Geometry check sheet. Reference: the model listing, model coordinates, mm. A direction names the side the tool comes from. Give positions to 0.01 mm unless a question says otherwise; leave off trailing zeros. Order: outer loops, then holes, each group sorted by start corner. A loop starts at its lowest first (then second) coordinate and runs counter-clockwise, first axis right, second up. Notation, with made-up numbers: M 34.5,-32.5 L 53.5,-32.5 A4 cw 53.5,-27.5 Z; hole C -31.75,67 d8. An arc over 180 degrees is marked long. Put each result on its own line as item: value. Start each with the question number.
Q1. Section check B-B on y = -62. Record the cut outline in (x, z).
Q2. Material ranges on L1, parallel to Y at x = -75.5, z = 34.5; L2, parallel to Z at x = -4, y = 32; L3, parallel to X at y = 14.5, z = 15.5, recorded low to high.
Q3. Go/stop test with flat-tipped pins: pin 1 (13.5 mm diameter, centred on x = -52.58, y = 8.41, fed in from +Z); pin 2 (2.5 mm diameter, centred on y = 37, z = 30.5, fed in from -X); pin 3 (3 mm diameter, centred on y = -52.5, z = 36, fed in from +X); pin 4 (19.5 mm diameter, centred on x = 89.5, y = -10, fed in from +Z). Record where each tip stops, or that it passes through.
Q4. Access from +Z, -Z, +X, -X, +Y, -Y to the whole of each face (thin tool, end or side, straight path). Record for faces 5 (the flat face through (-34, 31.909, 35)), 6 (the flat face through (-41.581, 18, 5)), 7 (the flat face through (49.547, -23.907, 4.93)).
Q5. Mould release check, pull along Y, two halves, no side actions. Record for faces 1 (the flat face through (74.71, -17.38, 34.65)), 2 (the flat face through (79.429, 5.975, 4.93)), 3 (the cylindrical face through (-44.474, 55.856, 4.93)), 4 (the flat face through (65.103, -39.463, 4.93)): +Y half, -Y half, draft (parallel to the pull), parting line (faces both ways), or undercut.
Q6. Section check A-A on z = 27. Record the cut outline in (x, y).
Autodesk Inventor part; units mm, degrees
ref_plane "YZ Plane" through (0, 0, 0) normal (1, 0, 0) x (0, 1, 0)
ref_plane "XZ Plane" through (0, 0, 0) normal (0, 1, 0) x (-1, 0, 0)
ref_plane "XY Plane" through (0, 0, 0) normal (0, 0, 1) x (1, 0, 0)
sketch "Sketch1" plane through (0, 0, 0) normal (0, 0, 1) x (1, 0, 0)
  line L0 (-127.5811, 34.9091) -> (-127.5811, 31.9091)
  line L1 (-127.5811, 34.9091) -> (-127.5811, 39.9091)
  line L2 (-127.5811, 31.9091) -> (-127.5811, 26.9091)
  line L3 (-127.5811, 26.9091) -> (19.1052, 26.9091)
  line L4 (-127.5811, 31.9091) -> (21.1763, 31.9091)
  line L5 (22.4189, 34.9091) -> (-127.5811, 34.9091)
  line L6 (24.49, 39.9091) -> (-127.5811, 39.9091)
  line L7 (126.3636, -73.2783) -> (21.1763, 31.9091)
  line L8 (22.4189, 34.9091) -> (128.4849, -71.157)
  line L9 (128.4849, -71.157) -> (126.3636, -73.2783)
  line L10 (19.1052, 26.9091) -> (126.3636, -80.3493)
  line L11 (135.556, -71.157) -> (24.49, 39.9091)
  line L12 (126.3636, -80.3493) -> (135.556, -71.157)
  line L13 (-87.5811, 26.9091) -> (-87.5811, 31.9091)
  line L14 (105.1971, 0.6309) -> (84.4826, -20.0836)
  circle A0 centre (97.4189, 8.4091) radius 8.5
  circle A1 centre (97.4189, 8.4091) radius 11
  line L15 (89.6407, 16.1872) -> (68.9263, -4.5272)
  line L16 (55.1971, -49.3691) -> (75.2902, -29.276)
  line L17 (39.6407, -33.8128) -> (59.7339, -13.7196)
  circle A2 centre (47.4189, -41.5909) radius 8.5
  circle A3 centre (47.4189, -41.5909) radius 11
  line L18 (-41.5811, 8.4091) -> (-41.5811, 26.9091)
  line L19 (-63.5811, 8.4091) -> (-63.5811, 26.9091)
  circle A4 centre (-52.5811, 8.4091) radius 8.5
  circle A5 centre (-52.5811, 8.4091) radius 11
  line L20 (-41.5811, 58.4091) -> (-41.5811, 39.9091)
  circle A6 centre (-52.5811, 58.4091) radius 8.5
  circle A7 centre (-52.5811, 58.4091) radius 11
  line L21 (-63.5811, 58.4091) -> (-63.5811, 39.9091)
  line L22 (-87.5811, 34.9091) -> (-87.5811, 39.9091)
  point P0 (0, 0)
  point P1 (-127.5811, 33.4091)
  point P2 (-127.5811, 33.4091)
  point P3 (-127.5811, 29.4091)
  point P4 (-87.5811, 29.4091)
  point P5 (-51.5456, 39.9091)
  dimension "d0" = 3
  dimension "d1" = 3
  dimension "d2" = 5
  dimension "d3" = 5
  dimension "d4" = 5
  dimension "d5" = 3
  dimension "d6" = 5
  dimension "d7" = 150
  dimension "d8" = 148.7574
  dimension "d9" = 148.7574
  dimension "d10" = 150
  dimension "d11" = 13
  dimension "d12" = 5
  dimension "d13" = 40
  dimension "d14" = 45
  dimension "d15" = 45
  dimension "d16" = 86
  dimension "d17" = 64
extrude "Extrusion1" add sketch "Sketch1" along normal blind 10 contours L5 L8 L9 L7 L4 L0 | L4 L13 L3 L2 | L21 A7 L20 L6 | L3 L18 A5 L19 | A7 | A5 | L15 A1 L14 L11 | L10 L16 A3 L17 | A1 | A3
extrude "Extrusion2" add sketch "Sketch1" along normal blind 60 contours L1 L6 L22 L5 | L22 L6 L11 L12 L10 L3 L13 L4 L7 L9 L8 L5
sketch "Sketch2" plane through (0, 0, 60) normal (0, 0, 1) x (1, 0, 0)
  line L0 (-127.5811, 39.9091) -> (-127.5811, 34.9091)
  line L1 (-127.5811, 34.9091) -> (22.4189, 34.9091)
  line L2 (-127.5811, 39.9091) -> (-87.5811, 39.9091)
  line L3 (-87.5811, 39.9091) -> (-87.5811, 34.9091)
  line L4 (-87.5811, 34.9091) -> (-127.5811, 34.9091)
  line L5 (-127.5811, 34.9091) -> (-127.5811, 39.9091)
  point P0 (0, 0)
  dimension "d22" = 40
extrude "Extrusion3" cut sketch "Sketch2" against normal blind 50
properties part number "hold_right"
Results found:
1. outline: M 108.01,0 L 126.4,0 L 126.4,60 L 119.33,60 L 119.33,10 L 115.09,10 L 115.09,60 L 108.01,60 Z
2. L1: y = 26.91 to 31.91, 34.91 to 39.91
2. L2: z = 0 to 10
2. L3: x = 31.51 to 38.59, 42.83 to 49.9
3. pin 1: passes through
3. pin 2: stops at x = -87.58
3. pin 3: stops at x = 118.4
3. pin 4: stops at z = 10
4. face 5: +Z, -X
4. face 6: +Z, -Z, -Y
4. face 7: +Z, -Z, -X
5. face 1: undercut
5. face 2: +Y half
5. face 3: undercut
5. face 4: -Y half
6. outline: M -87.58,26.91 L 19.11,26.91 L 126.36,-80.35 L 135.56,-71.16 L 24.49,39.91 L -87.58,39.91 L -87.58,34.91 L 22.42,34.91 L 128.48,-71.16 L 126.36,-73.28 L 21.18,31.91 L -87.58,31.91 Z
